from build123d import *

# Parameters (mm, degrees)
BOSS_EXTRUDE1_DEPTH      = 0.6
BOSS_EXTRUDE1_DEPTH_BACK = 0.6
SKETCH2_W                = 43.5
SKETCH2_H                = 15
BOSS_EXTRUDE2_DEPTH      = 2.8
BOSS_EXTRUDE2_DEPTH_BACK = 2.8
SKETCH3_W                = 30
SKETCH3_H                = 22
CUT_EXTRUDE1_DEPTH       = 53.980208569
CUT_EXTRUDE1_DEPTH_BACK  = 53.980208569
SKETCH4_R                = 2.25
SKETCH4_R_2              = 4


with BuildPart() as part:
    # Sketch2 → Boss-Extrude1 (new, two sides: drawn at the far end of the back side and taken through both)
    with BuildSketch(Plane(origin=(0, 0, 0), x_dir=(1, 0, 0), z_dir=(0, 1, 0)).offset(-BOSS_EXTRUDE1_DEPTH_BACK)):
        Rectangle(SKETCH2_W, SKETCH2_H)
    extrude(amount=BOSS_EXTRUDE1_DEPTH + BOSS_EXTRUDE1_DEPTH_BACK)

    # Sketch3 → Boss-Extrude2 (add, two sides: drawn at the far end of the back side and taken through both)
    with BuildSketch(Plane(origin=(0, 0, 0), x_dir=(1, 0, 0), z_dir=(0, 1, 0)).offset(-BOSS_EXTRUDE2_DEPTH_BACK)):
        with Locations((36.75, 0)):
            Rectangle(SKETCH3_W, SKETCH3_H)
        with Locations((-36.75, 0)):
            Rectangle(SKETCH3_W, SKETCH3_H)
    extrude(amount=BOSS_EXTRUDE2_DEPTH + BOSS_EXTRUDE2_DEPTH_BACK)

    # Sketch4 → Cut-Extrude1 (cut, two sides: drawn at the far end of the back side and taken through both)
    with BuildSketch(Plane(origin=(0, 0, 0), x_dir=(1, 0, 0), z_dir=(0, 1, 0)).offset(-CUT_EXTRUDE1_DEPTH_BACK)):
        with Locations(Location((28.25, 0, 0), (0, 0, 270))):
            Circle(SKETCH4_R)
        with Locations(Location((43.25, 0, 0), (0, 0, 270))):
            Circle(SKETCH4_R_2)
        with Locations(Location((-43.25, 0, 0), (0, 0, 90))):
            Circle(SKETCH4_R_2)
        with Locations(Location((-28.25, 0, 0), (0, 0, 90))):
            Circle(SKETCH4_R)
    extrude(amount=CUT_EXTRUDE1_DEPTH + CUT_EXTRUDE1_DEPTH_BACK, mode=Mode.SUBTRACT)


solid = part.part
Check sheet for the modelled part. Datum: model origin and axes. Units: mm. A direction names the side the tool comes from. Round coordinates to 2 decimals unless told otherwise and drop trailing zeros. Write each loop counter-clockwise with the first axis right and the second up, starting at its lowest first coordinate (ties: lowest second). Pieces come first, ordered by that corner, then holes. Notation, with made-up numbers: (88.25, 18) -> (134.25, 18) arc R11 cw to (134.25, 27) -> close; hole circle Ø5 at (67.5, 29.5). An arc over 180 degrees is marked (long way). Answer as CSV lines item,"result". Start each with the question number.
1) Go/stop test with flat-tipped pins: P1, Ø2.5, axis at x = 28.25, z = 0, coming from the +Y side; P2, Ø1, axis at x = 3.5, y = 0, coming from the -Z side; P3, Ø1.3, axis at x = 9, y = 0, coming from the +Z side; P4, Ø12, axis at x = -4.5, z = -3, coming from the -Y side. Record where each tip stops, or that it passes through.
2) Section check B-B on x = -43.25. Enter the section's corners in (y, z).
3) Section check C-C on x = -28.25. Enter the section's corners in (y, z).
4) Material ranges on line 1 (X direction, y = -0.85, z = 0); line 2 (X direction, y = 0.45, z = 0); line 3 (Z direction, x = 28.25, y = -0.65), recorded low to high. Write a range as from..to.
5) Tool access check on faces 1 (the flat face through (0, -0.6, 0)), 2 (the flat face through (0, 0.6, 0)), 3 (the cylindrical face through (47.216, -0.039, -0.521)). Record the directions out of +Z, -Z, +X, -X, +Y, -Y that give a thin tool (end or side, any length) a straight path to the whole face; none if there is none.
6) Section check D-D on x = -15. Enter the section's corners in (y, z).
7) Section check A-A on z = 0. Enter the section's corners in (x, y).
8) Release check for a two-part mould opening along X. For faces 4 (the flat face through (-51.75, 0, 0)), 5 (the flat face through (-37, 0, 11)), 6 (the cylindrical face through (-47.216, -0.039, 0.521)) record: pulls with the +X half, pulls with the -X half, needs draft (parallel to the pull), parting line crosses it, or undercut.
Found:
1,P1,"passes through"
1,P2,"stops at z = -7.5"
1,P3,"stops at z = 7.5"
1,P4,"stops at y = -0.6"
2,outline,"(-2.8, -11) -> (2.8, -11) -> (2.8, -4) -> (-2.8, -4) -> close; (-2.8, 4) -> (2.8, 4) -> (2.8, 11) -> (-2.8, 11) -> close"
3,outline,"(-2.8, -11) -> (2.8, -11) -> (2.8, -2.25) -> (-2.8, -2.25) -> close; (-2.8, 2.25) -> (2.8, 2.25) -> (2.8, 11) -> (-2.8, 11) -> close"
4,line 1,"x = -51.75..-47.25, -39.25..-30.5, -26..-21.75, 21.75..26, 30.5..39.25, 47.25..51.75"
4,line 2,"x = -51.75..-47.25, -39.25..-30.5, -26..26, 30.5..39.25, 47.25..51.75"
4,line 3,"z = -11..-2.25, 2.25..11"
5,face 1,"+Z, -Z, -Y"
5,face 2,"+Z, -Z, +Y"
5,face 3,"+Y, -Y"
6,outline,"(-0.6, -7.5) -> (0.6, -7.5) -> (0.6, 7.5) -> (-0.6, 7.5) -> close"
7,outline,"(-51.75, -2.8) -> (-47.25, -2.8) -> (-47.25, 2.8) -> (-51.75, 2.8) -> close; (-39.25, -2.8) -> (-30.5, -2.8) -> (-30.5, 2.8) -> (-39.25, 2.8) -> close; (-26, -2.8) -> (-21.75, -2.8) -> (-21.75, -0.6) -> (21.75, -0.6) -> (21.75, -2.8) -> (26, -2.8) -> (26, 2.8) -> (21.75, 2.8) -> (21.75, 0.6) -> (-21.75, 0.6) -> (-21.75, 2.8) -> (-26, 2.8) -> close; (30.5, -2.8) -> (39.25, -2.8) -> (39.25, 2.8) -> (30.5, 2.8) -> close; (47.25, -2.8) -> (51.75, -2.8) -> (51.75, 2.8) -> (47.25, 2.8) -> close"
8,face 4,"pulls with the -X half"
8,face 5,"needs draft"
8,face 6,"undercut"
